from build123d import *

# Parameters (mm, degrees)
CUT_EXTRUDE_1_DEPTH      = 107.939235082
CUT_EXTRUDE_1_DEPTH_BACK = 107.939235082
SKETCH_3_W               = 16
SKETCH_3_H               = 3.5
CUT_EXTRUDE_START        = 4.5
CUT_EXTRUDE_2_DEPTH      = 103.439235082
M5X0_8_1_D               = 4.2
M5X0_8_1_DEPTH           = 14
M5X0_8_1_CBORE_D         = 5
M5X0_8_1_CBORE_DEPTH     = 10
M5X0_8_1_TIP             = 1.2618073
CHAMFER_1_SIZE           = 1
CHAMFER_2_SIZE           = 0.5


with BuildPart() as part:
    # ｽｹｯﾁ5 → 回転1 (revolve)
    with BuildSketch(Plane.XY):
        Polygon((0, 0), (0, 7.5), (40.5, 7.5), (40.5, 7.2), (42, 7.2), (42, 10), (52, 10), (52, 7.2), (53.5, 7.2), (53.5, 7.5), (106, 7.5), (106, 0), align=None)
    revolve(axis=Axis((0, 0, 0), (-1, 0, 0)))

    # ｽｹｯﾁ3 → ｶｯﾄ - 押し出し1 (cut, two sides: drawn at the far end of the back side and taken through both)
    with BuildSketch(Plane.XY.offset(-CUT_EXTRUDE_1_DEPTH_BACK)):
        with Locations((8, 8.25)):
            Rectangle(SKETCH_3_W, SKETCH_3_H)
        with Locations((8, -8.25)):
            Rectangle(SKETCH_3_W, SKETCH_3_H)
    extrude(amount=CUT_EXTRUDE_1_DEPTH + CUT_EXTRUDE_1_DEPTH_BACK, mode=Mode.SUBTRACT)

    # ｽｹｯﾁ4 → ｶｯﾄ - 押し出し2 (cut, through all)
    with BuildSketch(Plane(origin=(0, 0, 0), x_dir=(1, 0, 0), z_dir=(0, 1, 0)).offset(CUT_EXTRUDE_START)):
        with BuildLine():
            Line((67.5, 2.5), (85.5, 2.5))
            ThreePointArc((85.5, 2.5), (88, 0), (85.5, -2.5))
            Line((85.5, -2.5), (67.5, -2.5))
            ThreePointArc((67.5, -2.5), (65, 0), (67.5, 2.5))
        make_face()
    extrude(amount=CUT_EXTRUDE_2_DEPTH, mode=Mode.SUBTRACT)

    # M5x0.8 ねじ穴1
    with Locations(Plane(origin=(0, 0, 0), x_dir=(0, -1, 0), z_dir=(-1, 0, 0))):
        with Locations((0, 0)):
            CounterBoreHole(M5X0_8_1_D / 2, M5X0_8_1_CBORE_D / 2, M5X0_8_1_CBORE_DEPTH, depth=M5X0_8_1_DEPTH)
            with Locations((0, 0, -(M5X0_8_1_DEPTH + M5X0_8_1_TIP / 2))):  # 118° drill point
                Cone(0, M5X0_8_1_D / 2, M5X0_8_1_TIP, mode=Mode.SUBTRACT)

    # 面取り1
    chamfer_1_edges = [part.edges().sort_by_distance(p)[0] for p in [
        (52, -10, 0),
        (42, -10, 0),
    ]]
    chamfer(chamfer_1_edges, length=CHAMFER_1_SIZE)

    # 面取り2
    chamfer_2_edges = [part.edges().sort_by_distance(p)[0] for p in [
        (0, 0, 7.5),
        (0, 0, -7.5),
        (106, -7.5, 0),
    ]]
    chamfer(chamfer_2_edges, length=CHAMFER_2_SIZE)


solid = part.part
Build history of the part. All positions in model axes, mm. A direction names the side the tool comes from. Give positions to 0.01 mm unless a question says otherwise; leave off trailing zeros. Order: outer loops, then holes, each group sorted by start corner. A loop starts at its lowest first (then second) coordinate and runs counter-clockwise, first axis right, second up. Notation, with made-up numbers: M -18.5,-1.5 L -3.5,-1.5 A5 ccw -3.5,3.5 Z; hole C 65.5,-30 d5. An arc over 180 degrees is marked long. Use one line per item in the form item = value.
1) Two-plate mould, pull along X, no slides. Class faces 6 (the face through (52.76, 6.87, -2.16)), 7 (the face through (15.04, -0.34, -0.14)), 8 (the face through (77, 4.5, 0)), 9 (the face through (20.78, -7.493, -0.33)): released by +X, released by -X, zero draft, split by the parting line, or undercut.
Calculated:
face_6 = undercut
face_7 = released by -X
face_8 = undercut
face_9 = zero draft
2) Saw through at A-A (x = 7). Give the cut face in (y, z).
Calculated:
outline = M -6.5,-3.74 A7.5 ccw 6.5,-3.74 L 6.5,3.74 A7.5 ccw -6.5,3.74 Z; hole C 0,0 d5
3) Saw through at B-B (x = 97). Give the cut face in (y, z), plus the area to 3 significant figures.
Calculated:
outline = C 0,0 d15
area = 177 mm2
4) Drop flat-ended pins along their axis: pin 1 (2 mm diameter, centred on x = 7, z = -0.5, fed in from -Y); pin 2 (2 mm diameter, centred on x = 80.5, y = 5.5, fed in from -Z); pin 3 (5 mm diameter, centred on x = 63, z = 1.5, fed in from +Y). Give the stop position or say it passes through.
Calculated:
pin_1 = -6.5
pin_2 = -6
pin_3 = 7.5
5) Tool access for faces 1 (the face through (8, -6.5, 0)), 2 (the face through (76, 6, -2.5)), 3 (the face through (52, 3, -7)), 4 (the face through (0, -3, 0)), 5 (the face through (8, 6.5, 0)): list every direction of +Z, -Z, +X, -X, +Y, -Y with a clear straight run to the whole face (end or side of a thin tool).
Calculated:
face_1 = +Z, -Z, -X, -Y
face_2 = +Y
face_3 = none
face_4 = +Z, -Z, -X, +Y, -Y
face_5 = +Z, -Z, -X, +Y
6) Probe probe 1 along Y at (x, z) = (12.7, 0); probe 2 along X at (y, z) = (-2, 7); probe 3 along Z at (x, y) = (6, 0). List the from-to ranges inside material, lowest first.
Calculated:
probe_1 = -6.5 to -2.1, 2.1 to 6.5
probe_2 = 0.28 to 40.5, 42 to 52, 53.5 to 105.72
probe_3 = -7.5 to -2.5, 2.5 to 7.5
